from build123d import *

# Parameters (mm, degrees)
SKETCH1_W           = 50
SKETCH1_H           = 25
BOSS_EXTRUDE1_DEPTH = 10
SKETCH2_W           = 20
SKETCH2_H           = 25
BOSS_EXTRUDE2_DEPTH = 75
SKETCH3_W           = 4
SKETCH3_H           = 25
CUT_EXTRUDE1_DEPTH  = 75
SKETCH4_R           = 1.966955022
CUT_EXTRUDE2_DEPTH  = 96.262794416
LPATTERN1_COUNT     = 7
LPATTERN1_PITCH     = 10
SKETCH5_W           = 15
SKETCH5_H           = 25
CUT_EXTRUDE3_DEPTH  = 94.541434669
SKETCH6_R           = 1.6
CUT_EXTRUDE4_DEPTH  = 96.262794416


with BuildPart() as part:
    # Sketch1 → Boss-Extrude1 (new body)
    with BuildSketch(Plane(origin=(0, 0, 0), x_dir=(1, 0, 0), z_dir=(0, 1, 0))):
        with Locations((25, 12.5)):
            Rectangle(SKETCH1_W, SKETCH1_H)
    extrude(amount=BOSS_EXTRUDE1_DEPTH)

    # Sketch2 → Boss-Extrude2 (add)
    with BuildSketch(Plane(origin=(0, 10, 0), x_dir=(1, 0, 0), z_dir=(0, 1, 0))):
        with Locations((25, 12.5)):
            Rectangle(SKETCH2_W, SKETCH2_H)
    extrude(amount=BOSS_EXTRUDE2_DEPTH)

    # Sketch3 → Cut-Extrude1 (cut)
    with BuildSketch(Plane(origin=(0, 85, 0), x_dir=(1, 0, 0), z_dir=(0, 1, 0))):
        with Locations((25, 12.5)):
            Rectangle(SKETCH3_W, SKETCH3_H)
    extrude(amount=-CUT_EXTRUDE1_DEPTH, mode=Mode.SUBTRACT)

    # Sketch4 → Cut-Extrude2 (cut, through all)
    with BuildSketch(Plane.ZY.offset(-15)):
        with Locations((-12.5, 80)):
            Circle(SKETCH4_R)
    cut_extrude2 = extrude(amount=-CUT_EXTRUDE2_DEPTH, mode=Mode.SUBTRACT)

    # LPattern1: Cut-Extrude2 ×7
    with Locations(*[(0, -i * LPATTERN1_PITCH, 0) for i in range(1, LPATTERN1_COUNT)]):
        add(cut_extrude2, mode=Mode.SUBTRACT)

    # Sketch5 → Cut-Extrude3 (cut, through all)
    with BuildSketch(Plane(origin=(0, 10, 0), x_dir=(1, 0, 0), z_dir=(0, 1, 0))):
        with Locations((42.5, 12.5)):
            Rectangle(SKETCH5_W, SKETCH5_H)
    extrude(amount=-CUT_EXTRUDE3_DEPTH, mode=Mode.SUBTRACT)

    # Sketch6 → Cut-Extrude4 (cut, through all)
    with BuildSketch(Plane.XZ):
        with Locations(Location((10.000440006, -19.069369087, 0), (0, 0, 270))):
            Circle(SKETCH6_R)
    cut_extrude4 = extrude(amount=-CUT_EXTRUDE4_DEPTH, mode=Mode.SUBTRACT)

    # Mirror1: Cut-Extrude4 across plane
    add(cut_extrude4.mirror(Plane.XY.offset(-12.5)), mode=Mode.SUBTRACT)


solid = part.part
Could you check a few things on this model? Use its own coordinates, in mm. A direction names the side the tool comes from. Coordinates: 2 decimals unless noted, no trailing zeros. Order: outer loops, then holes, each group sorted by start corner. A loop starts at its lowest first (then second) coordinate and runs counter-clockwise, first axis right, second up.
Q1. Suppose I cut it at A-A on y = 20. Please give me the cut outline in (x, z).
Q2. Thinking about a two-plate mould opening in X: for faces 4 (the flat face through (25, 10, -13)), 5 (the flat face through (35, 43, -12)), 6 (the flat face through (17, 0, -13)), which applies, released by +X, released by -X, zero draft, split by the parting line, or undercut?
Q3. Suppose I cut it at B-B on z = -2.75. Please give me the cut outline in (x, y).
Q4. Suppose I cut it at C-C on x = 29.5. Please give me the cut outline in (y, z), and give its area (3 significant figures).
Q5. Suppose I cut it at D-D on z = -19.5. Please give me the cut outline in (x, y).
Q6. Will these pins go through, and if not, where does the flat tip stop? pin 1 (3 mm diameter, centred on y = 60, z = -12.5, fed in from -X); pin 2 (2 mm diameter, centred on x = 25, z = -20.5, fed in from +Y); pin 3 (5 mm diameter, centred on y = 80, z = -12.5, fed in from -X).
Q7. Please list where these lines run through material, in increasing order: L1, parallel to X at y = 11.5, z = -17.25; L2, parallel to X at y = 5, z = -6; L3, parallel to Y at x = 13, z = -9.5.
Q8. Which directions (+Z, -Z, +X, -X, +Y, -Y) give clear straight access to the entire face, cutting with the end or side of a thin tool? Please do faces 1 (the flat face through (23, 48, -10)), 2 (the flat face through (15, 47, -12)), 3 (the cylindrical face through (30.94, 71.95, -12.76)).
Answer:
1. outline: (15, -25) - (23, -25) - (23, -14.47) - (15, -14.47) - close; (15, -10.53) - (23, -10.53) - (23, 0) - (15, 0) - close; (27, -25) - (35, -25) - (35, -14.47) - (27, -14.47) - close; (27, -10.53) - (35, -10.53) - (35, 0) - (27, 0) - close
2. face 4: undercut
2. face 5: released by +X
2. face 6: zero draft
3. outline: (0, 0) - (35, 0) - (35, 85) - (27, 85) - (27, 10) - (23, 10) - (23, 85) - (15, 85) - (15, 10) - (0, 10) - close
4. outline: (0, -25) - (85, -25) - (85, 0) - (0, 0) - close; hole circle Ø3.93 at (20, -12.5); hole circle Ø3.93 at (30, -12.5); hole circle Ø3.93 at (40, -12.5); hole circle Ø3.93 at (50, -12.5); hole circle Ø3.93 at (60, -12.5); hole circle Ø3.93 at (70, -12.5); hole circle Ø3.93 at (80, -12.5)
4. area: 2,040 mm2
5. outline: (0, 0) - (8.46, 0) - (8.46, 10) - (0, 10) - close; (11.54, 0) - (35, 0) - (35, 85) - (27, 85) - (27, 10) - (23, 10) - (23, 85) - (15, 85) - (15, 10) - (11.54, 10) - close
6. pin 1: passes through
6. pin 2: stops at y = 10
6. pin 3: stops at x = 15
7. L1: x = 15 to 23, 27 to 35
7. L2: x = 0 to 8.4, 11.6 to 35
7. L3: y = 0 to 10
8. face 1: +Z, -Z, +Y
8. face 2: +Z, -Z, -X, +Y
8. face 3: +X, -X
